Work out the finished part from the listing and answer in its coordinate system (mm). A direction names the side the tool comes from. Coordinates: 2 decimals unless noted, no trailing zeros. Order: outer loops, then holes, each group sorted by start corner. A loop starts at its lowest first (then second) coordinate and runs counter-clockwise, first axis right, second up. Notation, with made-up numbers: M 1,73.5 L 25,73.5 A17 ccw 25,87.5 Z; hole C 33,-19 d3. An arc over 180 degrees is marked long. Answer in a Markdown table with one row per item. Add a question column.
Item 1: The mould has two halves that part along Z. Classify faces 1 (the face through (-0.83, -260.44, 97.88)), 2 (the face through (28, -266.7, 28)), 3 (the face through (-127.192, -260.261, -40.055)): released by +Z, released by -Z, zero draft, split by the parting line, or undercut.
Item 2: The part is cut by section C-C (x = -101.6). Write down the section's boundary in (y, z).
Item 3: The part is cut by section D-D (z = -101.6). Write down the section's boundary in (x, y), then the cut area to 3 significant figures.
Item 4: Consider line 1 (Z direction, x = 0, y = -263) (3 decimals); line 2 (Y direction, x = 99, z = -6); line 3 (Z direction, x = 101.6, y = -257.25). Determine where each line is inside the solid, lowest interval first. Write a range as from..to.
Item 5: Which of the six approach directions +Z, -Z, +X, -X, +Y, -Y give full straight-line access (tool end or side, diameter ignored) to faces 4 (the face through (6.883, -183.172, 30.995)), 5 (the face through (6.883, -272.961, 30.995)), 6 (the face through (-0.83, -260.44, -105.32))?
Item 6: Flat-ended cylindrical pins translate along their axes: pin 1 Ø7 at (x, z) = (0, -101.6) entering from -Y; pin 2 Ø8 at (x, y) = (33, -194) entering from -Z; pin 3 Ø2.5 at (y, z) = (-233.5, 30.5) entering from +X; pin 4 Ø1 at (y, z) = (-230.5, 29.5) entering from -X. Find the tip coordinate at first contact, or state that the pin passes through.
Item 7: The part is cut by section A-A (z = 0). Write down the section's boundary in (x, y) (3 decimals).
Item 8: The part is cut by section B-B (x = 0). Write down the section's boundary in (y, z) (3 decimals), then the cut area to 3 significant figures.
from build123d import *

# Parameters (mm, degrees)
SKETCH2_R          = 28.575
CUT_EXTRUDE2_DEPTH = 228.6
CUT_EXTRUDE5_DEPTH = 8.89
SKETCH4_R          = 3.81
CUT_EXTRUDE4_DEPTH = 12.7


with BuildPart() as part:
    # Sketch1 → Revolve1 (revolve)
    with BuildSketch(Plane.XY, mode=Mode.PRIVATE) as revolve1_sk:
        Polygon((0, -114.3), (0, -279.4), (31.75, -279.4), (31.75, -266.7), (133.35, -266.7), (133.35, -254), (31.75, -254), (31.75, -114.3), align=None)
    revolve(revolve1_sk.sketch.rotate(Axis((0, 0, 0), (0, -1, 0)), 180), axis=Axis((0, 0, 0), (0, -1, 0)))

    # Sketch2 → Cut-Extrude2 (cut)
    with BuildSketch(Plane.XZ.offset(279.4)):
        Circle(SKETCH2_R)
    extrude(amount=-CUT_EXTRUDE2_DEPTH, mode=Mode.SUBTRACT)

    # Sketch3 → Cut-Extrude5 (cut)
    with BuildSketch(Plane.XY.offset(31.75)):
        Polygon((-6.35, -241.3), (6.35, -241.3), (6.35, -219.075), (0, -219.075), (-6.35, -219.075), align=None)
    extrude(amount=-CUT_EXTRUDE5_DEPTH, mode=Mode.SUBTRACT)

    # Sketch4 → Cut-Extrude4 (cut)
    with BuildSketch(Plane.XZ.offset(266.7)):
        with Locations((0, 101.6)):
            Circle(SKETCH4_R)
        with Locations((101.6, 0)):
            Circle(SKETCH4_R)
        with Locations((0, -101.6)):
            Circle(SKETCH4_R)
        with Locations((-101.6, 0)):
            Circle(SKETCH4_R)
    extrude(amount=-CUT_EXTRUDE4_DEPTH, mode=Mode.SUBTRACT)


solid = part.part
Reply:
| question | item | result |
|---|---|---|
| 1 | face 1 | undercut |
| 1 | face 2 | zero draft |
| 1 | face 3 | split by the parting line |
| 2 | outline | M -266.7,-86.37 L -254,-86.37 L -254,-3.81 L -266.7,-3.81 Z; M -266.7,3.81 L -254,3.81 L -254,86.37 L -266.7,86.37 Z |
| 3 | outline | M -86.37,-266.7 L -3.81,-266.7 L -3.81,-254 L -86.37,-254 Z; M 3.81,-266.7 L 86.37,-266.7 L 86.37,-254 L 3.81,-254 Z |
| 3 | area | 2,100 mm2 |
| 4 | line 1 | z = -133.35..-105.41, -97.79..-28.575, 28.575..97.79, 105.41..133.35 |
| 4 | line 2 | y = -266.7..-254 |
| 4 | line 3 | z = -86.37..-3.81, 3.81..86.37 |
| 5 | face 4 | +Y |
| 5 | face 5 | -Y |
| 5 | face 6 | +Y, -Y |
| 6 | pin 1 | passes through |
| 6 | pin 2 | stops at z = -12.93 |
| 6 | pin 3 | stops at x = 12.35 |
| 6 | pin 4 | stops at x = -12.93 |
| 7 | outline | M -133.35,-266.7 L -105.41,-266.7 L -105.41,-254 L -133.35,-254 Z; M -97.79,-266.7 L -31.75,-266.7 L -31.75,-279.4 L -28.575,-279.4 L -28.575,-114.3 L -31.75,-114.3 L -31.75,-254 L -97.79,-254 Z; M 28.575,-279.4 L 31.75,-279.4 L 31.75,-266.7 L 97.79,-266.7 L 97.79,-254 L 31.75,-254 L 31.75,-114.3 L 28.575,-114.3 Z; M 105.41,-266.7 L 133.35,-266.7 L 133.35,-254 L 105.41,-254 Z |
| 8 | outline | M -279.4,-31.75 L -266.7,-31.75 L -266.7,-97.79 L -254,-97.79 L -254,-31.75 L -114.3,-31.75 L -114.3,-28.575 L -279.4,-28.575 Z; M -279.4,28.575 L -241.3,28.575 L -241.3,31.75 L -254,31.75 L -254,97.79 L -266.7,97.79 L -266.7,31.75 L -279.4,31.75 Z; M -266.7,-133.35 L -254,-133.35 L -254,-105.41 L -266.7,-105.41 Z; M -266.7,105.41 L -254,105.41 L -254,133.35 L -266.7,133.35 Z; M -219.075,28.575 L -114.3,28.575 L -114.3,31.75 L -219.075,31.75 Z |
| 8 | area | 3,360 mm2 |
